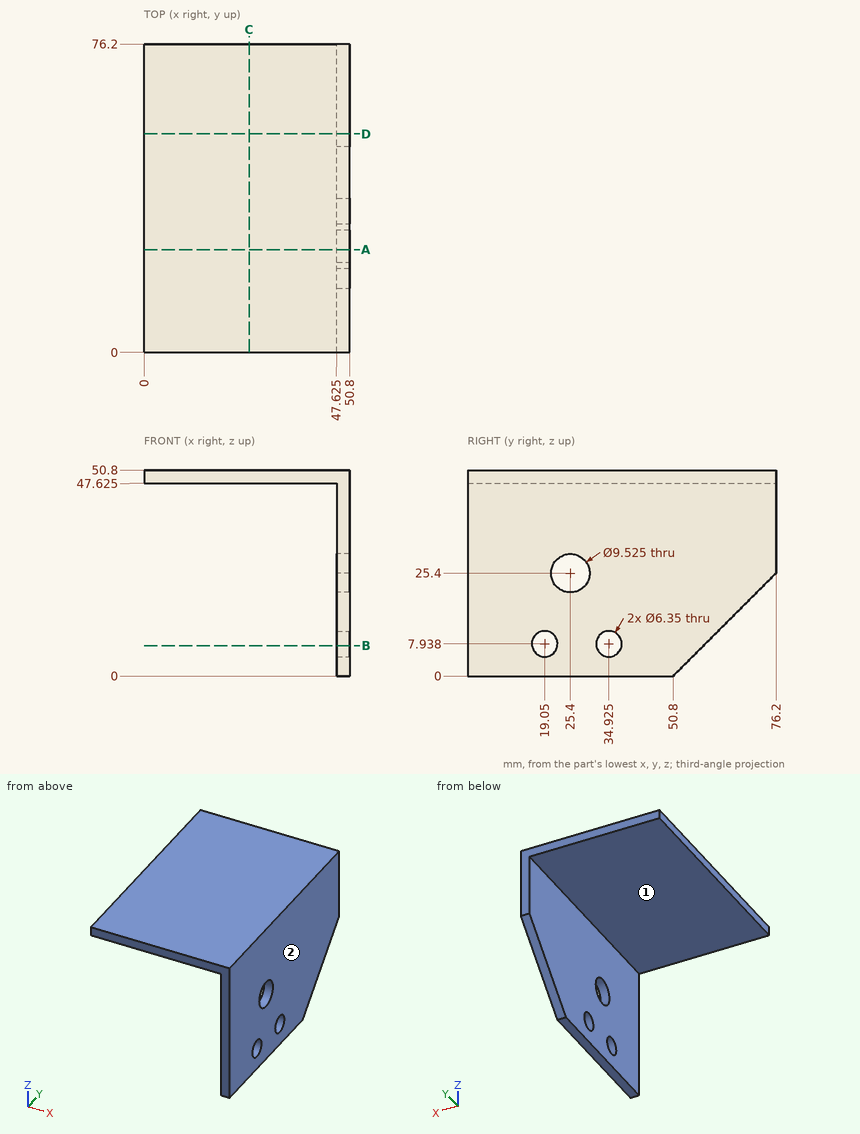
Source: three-view drawing plus pictorial views. Frame: mm from the lowest corner of the part. A direction names the side the tool comes from. Round coordinates to 2 decimals unless told otherwise and drop trailing zeros. Loops run counter-clockwise (first coordinate to the right, second up) from the corner with the lowest first, then second, coordinate; pieces in that order, holes last.
Q1. Pin query (flat end, axial travel): P1, Ø3, axis at x = 27, y = 27, coming from the -Z side (1 decimal); P2, Ø4, axis at y = 43, z = 18, coming from the -X side (1 decimal). Return the tip coordinate at first contact, or that it passes through.
Q2. Section B-B on z = 7.5. Return loops of the section in (x, y) (1 decimal).
Q3. Section A-A on y = 25.4. Return loops of the section in (x, z) (1 decimal).
Q4. Section D-D on y = 54. Return loops of the section in (x, z) (1 decimal).
Q5. Section C-C on x = 26. Return loops of the section in (y, z) (1 decimal).
Q6. Material intervals for L1, parallel to Z at x = 50.1, y = 19.05; L2, parallel to Z at x = 49.7, y = 25.4; L3, parallel to Z at x = 25, y = 14 (1 decimal), sorted ascending.
Q7. Access query for the marked faces 1 and 2. Directions: +Z, -Z, +X, -X, +Y, -Y. A direction counts if a zero-diameter tool reaches every point of the face in a straight line with its end or side. Return the directions, or none.
Evaluation:
1. P1: stops at z = 47.6
1. P2: stops at x = 47.6
2. outline: (47.6, 0) - (50.8, 0) - (50.8, 15.9) - (47.6, 15.9) - close; (47.6, 22.2) - (50.8, 22.2) - (50.8, 31.8) - (47.6, 31.8) - close; (47.6, 38.1) - (50.8, 38.1) - (50.8, 58.3) - (47.6, 58.3) - close
3. outline: (0, 47.6) - (47.6, 47.6) - (47.6, 30.2) - (50.8, 30.2) - (50.8, 50.8) - (0, 50.8) - close; (47.6, 0) - (50.8, 0) - (50.8, 20.6) - (47.6, 20.6) - close
4. outline: (0, 47.6) - (47.6, 47.6) - (47.6, 3.2) - (50.8, 3.2) - (50.8, 50.8) - (0, 50.8) - close
5. outline: (0, 47.6) - (76.2, 47.6) - (76.2, 50.8) - (0, 50.8) - close
6. L1: z = 0 to 4.76, 11.11 to 50.8
6. L2: z = 0 to 20.64, 30.16 to 50.8
6. L3: z = 47.6 to 50.8
7. face 1: -Z, -X, +Y, -Y
7. face 2: +Z, -Z, +X, +Y, -Y
